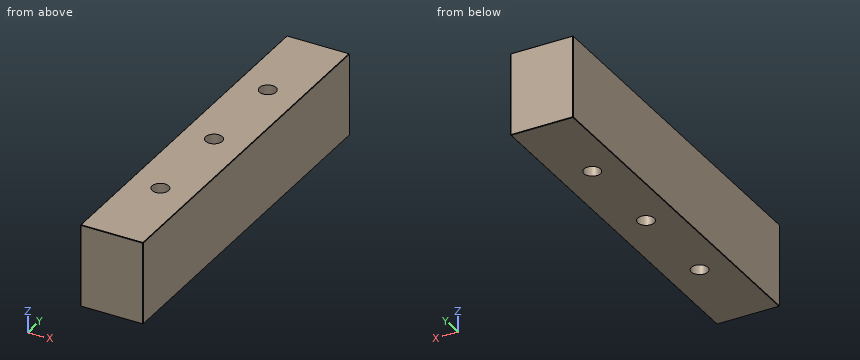
Autodesk Inventor part; units mm, degrees
ref_plane "Work Plane1" through (0, 0, 90) normal (0, 0, 1) x (1, 0, 0)
ref_plane "Work Plane2" through (0, 0, 0) normal (0, 0, -1) x (-1, 0, 0)
ref_plane "YZ Plane" through (0, 0, 0) normal (1, 0, 0) x (0, 1, 0)
sketch "Sketch1" plane through (0, 0, 0) normal (0, 0, 1) x (1, 0, 0)
  line L0 (-132, 200) -> (-200, 200)
  line L1 (-200, 200) -> (-200, -200)
  line L2 (-200, -200) -> (-132, -200)
  line L3 (-132, -200) -> (-132, 200)
  line L4 (200, 200) -> (200, -200)
  line L5 (132, -200) -> (132, 200)
  line L6 (132, 200) -> (200, 200)
  line L7 (132, -200) -> (200, -200)
  point P0 (0, 0)
  point P1 (-132, 0)
  point P2 (132, 0)
  point P3 (-165, 104)
  point P4 (165, 104)
  dimension "d85" = 400
  dimension "d86" = 68
  dimension "d88" = 68
  dimension "d89" = 200
  dimension "d93" = 400
  dimension "d94" = 200
  dimension "d98" = 104
  dimension "d100" = 165
  dimension "d101" = 165
  dimension "d102" = 104
extrude "Extrusion1" [suppressed]
extrude "Extrusion2" add sketch "Sketch1" along normal blind 90 contours L4 L7 L5 L6
hole "Hole1" [suppressed]
pattern_linear "Rectangular Pattern1" [suppressed]
hole "Hole2" at (165, 104, 0) direction (0, 0, 1) diameter 18 depth 90
pattern_linear "Rectangular Pattern2" count 3 spacing 104 along (0, -1, 0) of "Hole2"
ref_plane "Work Plane1" through (0, 0, 90) normal (0, 0, 1) x (1, 0, 0)
ref_plane "Work Plane2" through (0, 0, 0) normal (0, 0, -1) x (-1, 0, 0)
chamfer "Chamfer1" [suppressed]
chamfer "Chamfer2" distance 0.5 angle 45 12 edges at (132, 0, 90) (200, 0, 90) (166, -200, 90) (132, -200, 45) (200, -200, 45) (166, -200, 0) (200, 0, 0) (132, 0, 0) (200, 200, 45) (166, 200, 90) (132, 200, 45) (166, 200, 0)
equation "\"d85\" = L"
equation "\"d86\" = W_"
equation "\"d88\" = W_"
equation "\"d93\" = L"
equation "\"d20\" = H_"
equation "\"d95\" = H_"
equation "\"d129\" = S1_d1"
equation "\"d134\" = H_"
equation "\"d122\" = S1_d1"
equation "\"d127\" = H_"
properties part number "SA-SB-400x400x90" material "S 55 C"
Could you check a few things on this model? Use its own coordinates, in mm. Coordinates: 2 decimals unless noted, no trailing zeros. Write each loop counter-clockwise with the first axis right and the second up, starting at its lowest first coordinate (ties: lowest second). Pieces come first, ordered by that corner, then holes. Notation, with made-up numbers: (-14, 74.25) -> (-6, 74.25) arc R21 ccw to (-6, 90.25) -> close; hole circle Ø2 at (-38, 42). An arc over 180 degrees is marked (long way). Write item = value, one per line. Start each with the question number.
(1) I want a section at C-C (x = 160). Please give me the cut outline in (y, z).
(2) Will this pin go through, and if not, where does the flat tip stop? pin 1 (14.5 mm diameter, centred on x = 165, y = 0, fed in from -Z).
(3) I need wall thicknesses on line 1 (Y direction, x = 165, z = 20); line 2 (Y direction, x = 166, z = 29); line 3 (X direction, y = 104, z = 70). Which ranges of each line are inside material? Lowest first, please. Write a range as [from, to].
(4) I want a section at B-B (z = 54.5). Please give me the cut outline in (x, y), plus the area to 3 significant figures.
(5) I want a section at A-A (y = 104). Please give me the cut outline in (x, z).
Result set:
q1.outline = (-200, 0.5) -> (-199.5, 0) -> (-111.48, 0) -> (-111.48, 90) -> (-199.5, 90) -> (-200, 89.5) -> close; (-96.52, 0) -> (-7.48, 0) -> (-7.48, 90) -> (-96.52, 90) -> close; (7.48, 0) -> (96.52, 0) -> (96.52, 90) -> (7.48, 90) -> close; (111.48, 0) -> (199.5, 0) -> (200, 0.5) -> (200, 89.5) -> (199.5, 90) -> (111.48, 90) -> close
q2.pin_1 = through
q3.line_1 = [-200, -113], [-95, -9], [9, 95], [113, 200]
q3.line_2 = [-200, -112.94], [-95.06, -8.94], [8.94, 95.06], [112.94, 200]
q3.line_3 = [132, 156], [174, 200]
q4.outline = (132, -199.5) -> (132.5, -200) -> (199.5, -200) -> (200, -199.5) -> (200, 199.5) -> (199.5, 200) -> (132.5, 200) -> (132, 199.5) -> close; hole circle Ø18 at (165, -104); hole circle Ø18 at (165, 0); hole circle Ø18 at (165, 104)
q4.area = 26,400 mm2
q5.outline = (132, 0.5) -> (132.5, 0) -> (156, 0) -> (156, 90) -> (132.5, 90) -> (132, 89.5) -> close; (174, 0) -> (199.5, 0) -> (200, 0.5) -> (200, 89.5) -> (199.5, 90) -> (174, 90) -> close
